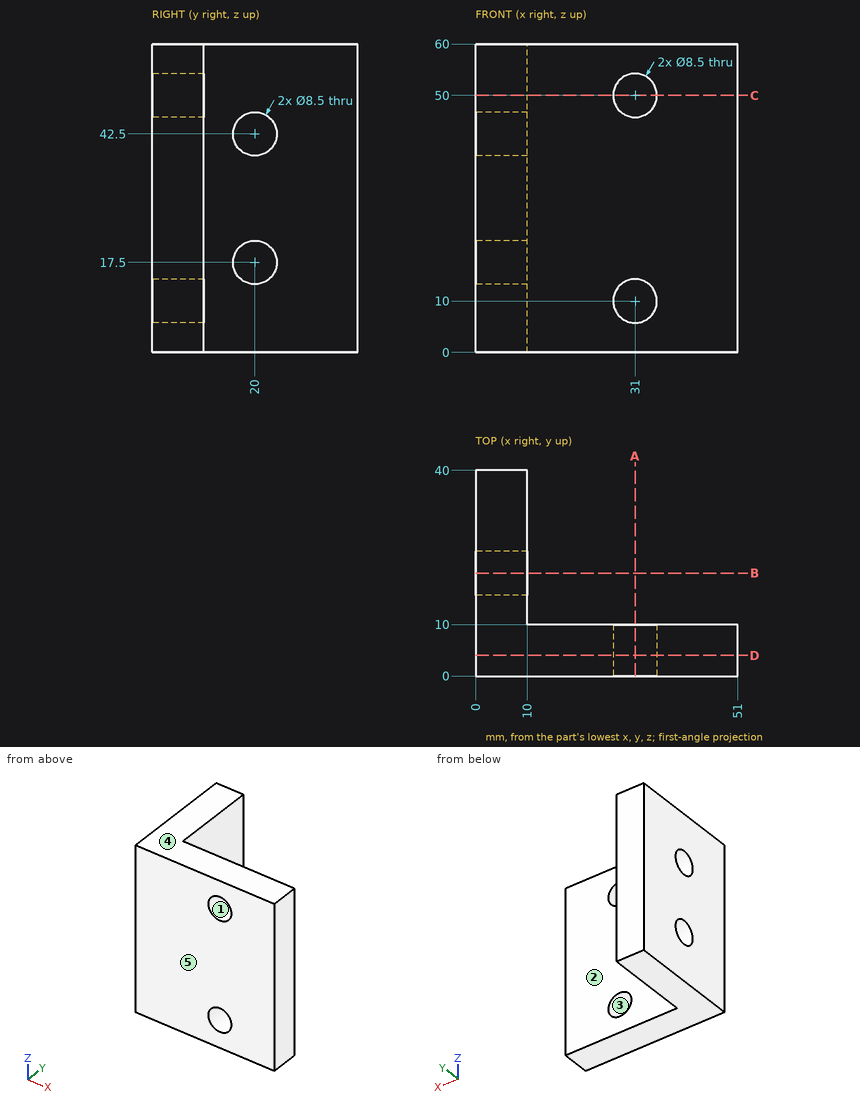
Design review of the part shown in the three views and the two pictorial views. Dimensions are in mm from the part's minimum x, y and z. A direction names the side the tool comes from. Round coordinates to 2 decimals unless told otherwise and drop trailing zeros. Loops run counter-clockwise (first coordinate to the right, second up) from the corner with the lowest first, then second, coordinate; pieces in that order, holes last. Notation, with made-up numbers: (10.5, 77.5) - (30.5, 77.5) arc R17 cw to (30.5, 83.5) - close; hole circle Ø9 at (-38.75, 1). An arc over 180 degrees is marked (long way). Write each question's results on one line, items separated by ' | '. Start each with the question number.
Q1. Take a section at D-D on y = 4. Give the boundary of the cut face in (x, z), plus the area to 3 significant figures.
Q2. Insertion check: P1, Ø6, axis at y = 16, z = 47, coming from the +X side; P2, Ø3, axis at x = 33, z = 26.5, coming from the +Y side. Each pin has a flat end and moves straight along its axis. Give the tip position at first contact, or say it passes through.
Q3. Take a section at C-C on z = 50. Give the boundary of the cut face in (x, y), plus the area to 3 significant figures.
Q4. Draft analysis for pull direction Z (two halves, no side actions). For the marked faces 3, 4 and 5, state which applies: pulls with the +Z half, pulls with the -Z half, needs draft (parallel to the pull), parting line crosses it, or undercut.
Q5. Take a section at B-B on y = 20. Give the boundary of the cut face in (x, z).
Q6. Wall thickness on line 1 along Z through (x, y) = (5, 20); line 2 along Y through (x, z) = (3, 17.5); line 3 along X through (y, z) = (8, 10): over which ranges is each line inside the solid? List them lowest first. Write a range as [from, to].
Q7. Tool access review of the marked faces 1 and 2: name each direction out of +Z, -Z, +X, -X, +Y, -Y from which nothing blocks a thin tool from reaching the whole face with its end or side.
Q8. Take a section at A-A on x = 31. Give the boundary of the cut face in (y, z).
Data:
1) outline: (0, 0) - (51, 0) - (51, 60) - (0, 60) - close; hole circle Ø8.5 at (31, 10); hole circle Ø8.5 at (31, 50) | area: 2,950 mm²
2) P1: stops at x = 10 | P2: stops at y = 10
3) outline: (0, 0) - (26.75, 0) - (26.75, 10) - (10, 10) - (10, 40) - (0, 40) - close; (35.25, 0) - (51, 0) - (51, 10) - (35.25, 10) - close | area: 725 mm²
4) face 3: undercut | face 4: pulls with the +Z half | face 5: needs draft
5) outline: (0, 0) - (10, 0) - (10, 13.25) - (0, 13.25) - close; (0, 21.75) - (10, 21.75) - (10, 38.25) - (0, 38.25) - close; (0, 46.75) - (10, 46.75) - (10, 60) - (0, 60) - close
6) line 1: z = [0, 13.25], [21.75, 38.25], [46.75, 60] | line 2: y = [0, 15.75], [24.25, 40] | line 3: x = [0, 26.75], [35.25, 51]
7) face 1: +Y, -Y | face 2: +Z, -Z, +X, +Y
8) outline: (0, 0) - (10, 0) - (10, 5.75) - (0, 5.75) - close; (0, 14.25) - (10, 14.25) - (10, 45.75) - (0, 45.75) - close; (0, 54.25) - (10, 54.25) - (10, 60) - (0, 60) - close
